CAD build for the part. Positions are in the model's coordinates, mm. A direction names the side the tool comes from. Coordinates: 2 decimals unless noted, no trailing zeros. Loops run counter-clockwise (first coordinate to the right, second up) from the corner with the lowest first, then second, coordinate; pieces in that order, holes last. Notation, with made-up numbers: (-4.5, -3) -> (35.5, -3) arc R22 ccw to (35.5, 15) -> close; hole circle Ø3 at (-31.75, -13). An arc over 180 degrees is marked (long way). Write item = value, one per line. Start each with the question number.
(1) Band-saw the part on A-A (y = 0). Write the cut outline in (x, z), and give its area (3 significant figures).
(2) Band-saw the part on D-D (x = 26). Write the cut outline in (y, z).
(3) Pull direction Y, two halves, no side cores. Call faces 1 (the face through (24.409, 3.905, -0.867)), 2 (the face through (18, -4.3, 0.1)), 3 (the face through (9.9, 0, 0)): +Y half, -Y half, draft (parallel to the pull), parting line (faces both ways), or undercut.
(4) Tool access for faces 4 (the face through (15.979, -8.872, -4.614)), 5 (the face through (31, 0, 0)): list every direction of +Z, -Z, +X, -X, +Y, -Y with a clear straight run to the whole face (end or side of a thin tool).
(5) Flat gauge pins, fed straight in: P1, Ø8, axis at x = -13, z = 7, coming from the -Y side; P2, Ø10, axis at x = 10, y = -0.5, coming from the -Z side; P3, Ø6, axis at x = 2.5, y = 8.5, coming from the -Z side; P4, Ø11.5, axis at y = -1, z = -3, coming from the -X side. Where does each tip first touch, or does it go through?
(6) Band-saw the part on B-B (z = -1.75). Write the cut outline in (x, y), and give its area (3 significant figures).
(7) Band-saw the part on C-C (x = 0). Write the cut outline in (y, z), and give its area (3 significant figures).
(8) Drill centre lines: line 1 (Y direction, x = 7, z = 2.25); line 2 (X direction, y = 4, z = -0.5); line 3 (X direction, y = -7, z = 2.75). Where is each one in solid material? Low to high. Write a range as from..to.
```python
from build123d import *

# Parameters (mm, degrees)
IZIM2_R                     = 4
Y_KSEKLIK_EKSTR_ZYON1_START = 18
IZIM4_R                     = 10
Y_KSEKLIK_EKSTR_ZYON1_DEPTH = 8.1
PAH1_SIZE                   = 4
IZIM6_R                     = 4
Y_KSEKLIK_EKSTR_ZYON2_DEPTH = 13


with BuildPart() as part:
    # Süpür1: sweep along a path in Çizim1
    with BuildLine(Plane.XY) as s_p_r1_path:
        CenterArc((0, 0), 14, 0, 360)
    # Çizim2 → Süpür1 (sweep)
    with BuildSketch(Plane(origin=(0, 0, 0), x_dir=(1, 0, 0), z_dir=(0, 1, 0))):
        with Locations((14, 0)):
            Circle(IZIM2_R)
    sweep(path=s_p_r1_path.line)

    # Çizim4 → Yükseklik-Ekstrüzyon1 (add)
    with BuildSketch(Plane(origin=(0, 0, 0), x_dir=(0, 0, -1), z_dir=(1, 0, 0)).offset(Y_KSEKLIK_EKSTR_ZYON1_START)):
        Circle(IZIM4_R)
    extrude(amount=-Y_KSEKLIK_EKSTR_ZYON1_DEPTH)

    # Pah1
    pah1_edges = [part.edges().sort_by_distance(p)[0] for p in [
        (9.9, 0, 10),
        (9.9, 5.491506193, -8.357233976),
    ]]
    chamfer(pah1_edges, length=PAH1_SIZE)

    # Çizim6 → Yükseklik-Ekstrüzyon2 (add)
    with BuildSketch(Plane(origin=(18, 0, 0), x_dir=(0, 0, -1), z_dir=(1, 0, 0))):
        with Locations(Location((0, 0, 0), (0, 0, 180))):
            Circle(IZIM6_R)
    extrude(amount=Y_KSEKLIK_EKSTR_ZYON2_DEPTH)


solid = part.part
```
Findings below:
q1.outline = circle Ø8 at (-14, 0); (9.9, -6) -> (13.9, -10) -> (18, -10) -> (18, -4) -> (31, -4) -> (31, 4) -> (18, 4) -> (18, 10) -> (13.9, 10) -> (9.9, 6) -> close
q1.area = 300 mm²
q2.outline = circle Ø8 at (0, 0)
q3.face_1 = parting line
q3.face_2 = draft
q3.face_3 = undercut
q4.face_4 = +X
q4.face_5 = +Z, -Z, +X, +Y, -Y
q5.P1 = -11.53
q5.P2 = -10
q5.P3 = -3.38
q5.P4 = -18
q6.outline = (14.58, -9.85) -> (18, -9.85) -> (18, -3.6) -> (31, -3.6) -> (31, 3.6) -> (18, 3.6) -> (18, 9.85) -> (14.58, 9.85) arc R17.6 ccw (long way) to start; hole (9.9, -3.2) -> (9.9, 3.2) arc R10.4 ccw (long way) to start
q6.area = 755 mm²
q7.outline = circle Ø8 at (-14, 0); circle Ø8 at (14, 0)
q7.area = 101 mm²
q8.line_1 = -15.83..-8.08, 8.08..15.83
q8.line_2 = -17.52..-9.2, 9.2..18
q8.line_3 = -15.39..-8.61, 8.61..18
